The model under review builds one solid part; all positions refer to its coordinate system, in mm. A direction names the side the tool comes from. Coordinates: 2 decimals unless noted, no trailing zeros. Order: outer loops, then holes, each group sorted by start corner. A loop starts at its lowest first (then second) coordinate and runs counter-clockwise, first axis right, second up.
Autodesk Inventor part; units mm, degrees
ref_plane "YZ Plane" through (0, 0, 0) normal (1, 0, 0) x (0, 1, 0)
ref_plane "XZ Plane" through (0, 0, 0) normal (0, 1, 0) x (-1, 0, 0)
ref_plane "XY Plane" through (0, 0, 0) normal (0, 0, 1) x (1, 0, 0)
sketch "Sketch1" plane through (0, 0, 0) normal (0, 0, 1) x (1, 0, 0)
  line L0 (0, 0) -> (0, 88.9) construction
  circle A0 centre (0, 88.9) radius 6.35
  arc A1 (8.9901, 92.0471) -> (-8.9901, 92.0471) centre (0, 88.9) ccw
  line L1 (0, 0) -> (-38.1, 0)
  line L2 (-38.1, 0) -> (-38.1, 8.89)
  line L3 (-38.1, 8.89) -> (-8.9901, 92.0471)
  line L4 (0, 0) -> (38.1, 0)
  line L5 (38.1, 0) -> (38.1, 8.89)
  line L6 (38.1, 8.89) -> (8.9901, 92.0471)
  line L7 (-20.9396, 38.6924) -> (-28.6314, 16.7194)
  line L8 (-20.9396, 12.7) -> (0, 12.7) construction
  arc A2 (-29.5978, 13.9588) -> (-26.0017, 8.89) centre (-26.0017, 12.7) ccw
  line L9 (-28.6314, 16.7194) -> (-29.5978, 13.9588)
  line L10 (-20.9396, 8.89) -> (-26.0017, 8.89)
  line L11 (-20.9396, 12.7) -> (-26.0017, 12.7) construction
  circle A3 centre (0, 12.7) radius 3.81 construction
  arc A4 (-7.62, 8.89) -> (-3.81, 12.7) centre (-7.62, 12.7) ccw
  line L12 (-3.81, 12.7) -> (-3.81, 43.5601)
  line L13 (-26.0017, 12.7) -> (-13.8789, 47.3309) construction
  line L14 (-23.545, 50.4685) -> (0, 42.2264) construction
  line L15 (-24.8039, 46.8725) -> (0, 38.1897) construction
  line L16 (-20.9396, 38.6924) -> (-18.8105, 44.7745)
  line L17 (-15.2144, 43.5156) -> (-3.81, 43.5601) construction
  circle A5 centre (-3.81, 43.5601) radius 3.81 construction
  line L18 (-7.6348, 47.3552) -> (-15.2293, 47.3256)
  arc A6 (-15.2293, 47.3256) -> (-18.8105, 44.7745) centre (-15.2144, 43.5156) ccw
  arc A7 (-3.81, 43.5304) -> (-7.6348, 47.3552) centre (-7.62, 43.5452) ccw
  line L19 (-20.9396, 8.89) -> (-7.62, 8.89)
  line L20 (20.9396, 38.6924) -> (28.6314, 16.7194)
  arc A8 (26.0017, 8.89) -> (29.5978, 13.9588) centre (26.0017, 12.7) ccw
  line L21 (20.9396, 8.89) -> (26.0017, 8.89)
  arc A9 (3.81, 12.7) -> (7.62, 8.89) centre (7.62, 12.7) ccw
  line L22 (3.81, 12.7) -> (3.81, 43.5601)
  line L23 (20.9396, 38.6924) -> (18.8105, 44.7745)
  line L24 (7.6348, 47.3552) -> (15.2293, 47.3256)
  arc A10 (18.8105, 44.7745) -> (15.2293, 47.3256) centre (15.2144, 43.5156) ccw
  arc A11 (7.6348, 47.3552) -> (3.81, 43.5304) centre (7.62, 43.5452) ccw
  line L25 (20.9396, 8.89) -> (7.62, 8.89)
  line L26 (28.6314, 16.7194) -> (29.5978, 13.9588)
  point P0 (-3.81, 64.5628)
  dimension "d20" = 7.62
  dimension "d0" = 88.9
  dimension "d2" = 12.7
  dimension "d3" = 19.05
  dimension "d5" = 38.1
  dimension "d6" = 90
  dimension "d7" = 8.89
  dimension "d14" = 6.35
  dimension "d16" = 7.62
  dimension "d17" = 70.707
  dimension "d18" = 3.81
  dimension "d22" = 3.81
  dimension "d23" = 3.81
  dimension "d24" = 12.7
  dimension "d25" = 3.81
extrude "Extrusion1" add sketch "Sketch1" along normal mid plane 12.7
sketch "Sketch2" plane through (0, 0, 6.35) normal (0, 0, 1) x (1, 0, 0)
  arc A0 (26.0017, 8.89) -> (29.5978, 13.9588) centre (26.0017, 12.7) ccw
  line L0 (26.0017, 8.89) -> (7.62, 8.89)
  arc A1 (3.81, 12.7) -> (7.62, 8.89) centre (7.62, 12.7) ccw
  line L1 (3.81, 12.7) -> (3.81, 43.5304)
  arc A2 (7.6348, 47.3552) -> (3.81, 43.5304) centre (7.62, 43.5452) ccw
  line L2 (7.6348, 47.3552) -> (15.2293, 47.3256)
  arc A3 (18.8105, 44.7745) -> (15.2293, 47.3256) centre (15.2144, 43.5156) ccw
  line L3 (18.8105, 44.7745) -> (29.5978, 13.9588)
  arc A4 (-15.2293, 47.3256) -> (-18.8105, 44.7745) centre (-15.2144, 43.5156) ccw
  line L4 (-15.2293, 47.3256) -> (-7.6348, 47.3552)
  arc A5 (-3.81, 43.5304) -> (-7.6348, 47.3552) centre (-7.62, 43.5452) ccw
  line L5 (-3.81, 43.5304) -> (-3.81, 12.7)
  arc A6 (-7.62, 8.89) -> (-3.81, 12.7) centre (-7.62, 12.7) ccw
  line L6 (-7.62, 8.89) -> (-26.0017, 8.89)
  arc A7 (-29.5978, 13.9588) -> (-26.0017, 8.89) centre (-26.0017, 12.7) ccw
  line L7 (-29.5978, 13.9588) -> (-18.8105, 44.7745)
  circle A8 centre (0, 88.9) radius 6.35
  line L8 (-38.1, 0) -> (38.1, 0)
  line L9 (38.1, 0) -> (38.1, 8.89)
  line L10 (38.1, 8.89) -> (8.9901, 92.0471)
  arc A9 (8.9901, 92.0471) -> (-8.9901, 92.0471) centre (0, 88.9) ccw
  line L11 (-8.9901, 92.0471) -> (-38.1, 8.89)
  line L12 (-38.1, 8.89) -> (-38.1, 0)
  point P0 (0, 0)
sketch "Sketch3" plane through (0, 0, 6.35) normal (0, 0, 1) x (1, 0, 0)
  line L0 (-38.1, 0) -> (38.1, 0)
  line L1 (38.1, 0) -> (38.1, 8.89)
  line L2 (-38.1, 0) -> (38.1, 0)
  line L3 (38.1, 0) -> (38.1, 8.89)
  line L4 (38.1, 8.89) -> (-38.1, 8.89)
  line L5 (-38.1, 8.89) -> (-38.1, 0)
  point P0 (0, 0)
extrude "Extrusion2" add sketch "Sketch3" along normal blind 6.35
mirror "Mirror1" about plane through (0, 0, 0) normal (0, 0, 1) of "Extrusion2"
properties part number "Y_axis_shaft_end_support" material "Aluminum 6061"
(1) Wall thickness on line 1 (Y direction, x = 0, z = 3); line 2 (X direction, y = 36, z = 5); line 3 (Z direction, x = 0.5, y = 29.5): over which ranges is each line inside the solid? List them lowest first.
(2) Consider section B-B (z = 4.75). Give the boundary of the cut face in (x, y), then the cut area to 3 significant figures.
(3) Consider section C-C (y = 88.9). Give the boundary of the cut face in (x, z).
(4) Tool access review of faces 1 (the face through (0, 51, 6.35)), 2 (the face through (29.14, 10.54, -0.09)), 3 (the face through (38.1, 5, 0)): name each direction out of +Z, -Z, +X, -X, +Y, -Y from which nothing blocks a thin tool from reaching the whole face with its end or side.
(5) Insertion check: pin 1 Ø23 at (x, y) = (1.5, 33.5) entering from -Z; pin 2 Ø4 at (y, z) = (25, 0.5) entering from -X; pin 3 Ø10 at (x, y) = (-14.5, 70) entering from +Z. Each pin has a flat end and moves straight along its axis. Give the tip position at first contact, or say it passes through.
(6) Consider section D-D (y = 22.5). Give the boundary of the cut face in (x, z), then the cut area to 3 significant figures.
(7) Consider section A-A (x = 0). Give the boundary of the cut face in (y, z), then the cut area to 3 significant figures.
Findings:
1. line 1: y = 0 to 82.55, 95.25 to 98.43
1. line 2: x = -28.61 to -21.88, -3.81 to 3.81, 21.88 to 28.61
1. line 3: z = -6.35 to 6.35
2. outline: (-38.1, 0) - (38.1, 0) - (38.1, 8.89) - (8.99, 92.05) arc R9.53 ccw to (-8.99, 92.05) - (-38.1, 8.89) - close; hole (-29.6, 13.96) arc R3.81 ccw to (-26, 8.89) - (-7.62, 8.89) arc R3.81 ccw to (-3.81, 12.7) - (-3.81, 43.56) arc R3.81 ccw to (-7.63, 47.36) - (-15.23, 47.33) arc R3.81 ccw to (-18.81, 44.77) - (-20.94, 38.69) - (-28.63, 16.72) - close; hole circle Ø12.7 at (0, 88.9); hole (3.81, 12.7) arc R3.81 ccw to (7.62, 8.89) - (26, 8.89) arc R3.81 ccw to (29.6, 13.96) - (28.63, 16.72) - (20.94, 38.69) - (18.81, 44.77) arc R3.81 ccw to (15.23, 47.33) - (7.63, 47.36) arc R3.81 ccw to (3.81, 43.56) - close
2. area: 2,980 mm2
3. outline: (-10.09, -6.35) - (-6.35, -6.35) - (-6.35, 6.35) - (-10.09, 6.35) - close; (6.35, -6.35) - (10.09, -6.35) - (10.09, 6.35) - (6.35, 6.35) - close
4. face 1: +Z, +X, -X, +Y
4. face 2: +Z, -Z
4. face 3: +Z, -Z, +X, +Y, -Y
5. pin 1: stops at z = -6.35
5. pin 2: stops at x = -33.16
5. pin 3: stops at z = 6.35
6. outline: (-33.34, -6.35) - (-26.61, -6.35) - (-26.61, 6.35) - (-33.34, 6.35) - close; (-3.81, -6.35) - (3.81, -6.35) - (3.81, 6.35) - (-3.81, 6.35) - close; (26.61, -6.35) - (33.34, -6.35) - (33.34, 6.35) - (26.61, 6.35) - close
6. area: 268 mm2
7. outline: (0, -12.7) - (8.89, -12.7) - (8.89, -6.35) - (82.55, -6.35) - (82.55, 6.35) - (8.89, 6.35) - (8.89, 12.7) - (0, 12.7) - close; (95.25, -6.35) - (98.43, -6.35) - (98.43, 6.35) - (95.25, 6.35) - close
7. area: 1,200 mm2
